Autodesk Inventor part; units mm, degrees
ref_plane "YZ Plane" through (0, 0, 0) normal (1, 0, 0) x (0, 1, 0)
ref_plane "XZ Plane" through (0, 0, 0) normal (0, 1, 0) x (-1, 0, 0)
ref_plane "XY Plane" through (0, 0, 0) normal (0, 0, 1) x (1, 0, 0)
sketch "Sketch1" plane through (0, 0, 0) normal (0, 1, 0) x (-1, 0, 0)
  line L0 (0, 0) -> (-21, 0)
  line L1 (-21, 0) -> (-21, -14)
  line L2 (-21, -14) -> (0, -14)
  line L3 (0, -14) -> (0, 0)
  dimension "d0" = 21
  dimension "d1" = 14
extrude "Extrusion1" add sketch "Sketch1" along normal blind 1.7
sketch "Sketch2" plane through (0, 0, 0) normal (0, -1, 0) x (1, 0, 0)
  line L0 (0, 0) -> (21, 0)
  line L1 (0, -14) -> (0, 0)
  line L2 (-4.6, 0) -> (27.6, 0)
  line L3 (0, -16.8) -> (0, 2.8)
  line L4 (0.52, -0.17) -> (6.02, -0.17)
  line L5 (6.02, -0.17) -> (6.02, -13.67)
  line L6 (6.02, -13.67) -> (0.52, -13.67)
  line L7 (0.52, -13.67) -> (0.52, -0.17)
  line L8 (2, -1.84) -> (2, -0.17)
  line L9 (2, -1.84) -> (0.52, -1.84)
  line L10 (4.54, -12) -> (4.54, -13.67)
  line L11 (4.54, -12) -> (6.02, -12)
  point P0 (4.54, -1.84)
  point P1 (2, -4.38)
  point P2 (4.54, -4.38)
  point P3 (2, -6.92)
  point P4 (4.54, -6.92)
  point P5 (2, -9.46)
  point P6 (4.54, -9.46)
  point P7 (2, -12)
  dimension "d12" = 2.54
  dimension "d15" = 2.54
  dimension "d18" = 5.5
  dimension "d19" = 13.5
  dimension "d20" = 4.38
  dimension "d21" = 4.54
extrude "Extrusion2" add sketch "Sketch2" along normal blind 9
sketch "Sketch3" plane through (0, 0, 0) normal (0, -1, 0) x (1, 0, 0)
  line L0 (0, -14) -> (0, 0)
  line L1 (13.1877, -8.8011) -> (20.6877, -8.8011)
  line L2 (20.6877, -8.8011) -> (20.6877, -0.3011)
  line L3 (20.6877, -0.3011) -> (13.1877, -0.3011)
  line L4 (13.1877, -0.3011) -> (13.1877, -8.8011)
  line L5 (19.1, -2.8011) -> (19.1, -0.3011)
  line L6 (19.1, -6.3011) -> (19.1, -8.8011)
  dimension "d25" = 19.1
  dimension "d26" = 3.5
  dimension "d27" = 7.5
  dimension "d28" = 8.5
extrude "Extrusion3" add sketch "Sketch3" along normal blind 13
properties part number "ccpad"
Design review of the part built by this model. Coordinates are the model's own, in mm. A direction names the side the tool comes from. Coordinates: 2 decimals unless noted, no trailing zeros. Write each loop counter-clockwise with the first axis right and the second up, starting at its lowest first coordinate (ties: lowest second). Pieces come first, ordered by that corner, then holes. Notation, with made-up numbers: M 41.25,46 L 99.25,46 A19 cw 99.25,57 Z; hole C 20,-6.5 d2. An arc over 180 degrees is marked long. Answer as a JSON object with one key per item and string values.
Item 1: Add section A-A, the plane y = -5.75. Give the boundary of the cut face in (x, z), and give its area (3 significant figures).
Outcome:
{"outline": "M 0.52,-13.67 L 6.02,-13.67 L 6.02,-0.17 L 0.52,-0.17 Z; M 13.19,-8.8 L 20.69,-8.8 L 20.69,-0.3 L 13.19,-0.3 Z", "area": "138 mm²"}
Item 2: Insertion check: pin 1 Ø2 at (y, z) = (-5, -5.5) entering from +X; pin 2 Ø1.5 at (x, z) = (3.5, -3.5) entering from -Y; pin 3 Ø2 at (x, y) = (15.5, -6) entering from -Z. Each pin has a flat end and moves straight along its axis. Give the tip position at first contact, or say it passes through.
Outcome:
{"pin 1": "x = 20.69", "pin 2": "y = -9", "pin 3": "z = -8.8"}
Item 3: Wall thickness on probe 1 along X at (y, z) = (-4.75, -6.5); probe 2 along Y at (x, z) = (3.75, -2); probe 3 along Z at (x, y) = (5.5, -3): over which ranges is each line inside the solid? List them lowest first.
Outcome:
{"probe 1": "0.52 to 6.02, 13.19 to 20.69", "probe 2": "-9 to 1.7", "probe 3": "-13.67 to -0.17"}
Item 4: Add section D-D, the plane z = -0.75. Give the boundary of the cut face in (x, y), and give its area (3 significant figures).
Outcome:
{"outline": "M 0,0 L 0.52,0 L 0.52,-9 L 6.02,-9 L 6.02,0 L 13.19,0 L 13.19,-13 L 20.69,-13 L 20.69,0 L 21,0 L 21,1.7 L 0,1.7 Z", "area": "183 mm²"}
Item 5: Machinability: for faces 5 (the flat face through (3, -4, -0.17)), 6 (the flat face through (13.188, -6, -4)), 7 (the flat face through (0.52, -4, -7)), 8 (the flat face through (17, -6, -8.801)), which of the approach directions +Z, -Z, +X, -X, +Y, -Y give a long, thin tool a straight path to every point of the face, cutting with its end or side? Answer none if there is none.
Outcome:
{"face 5": "+Z, +X, -X, -Y", "face 6": "+Z, -Z, -Y", "face 7": "+Z, -Z, -X, -Y", "face 8": "-Z, +X, -Y"}
Item 6: Draft analysis for pull direction X (two halves, no side actions). For faces 1 (the flat face through (6.02, -4, -7)), 2 (the flat face through (21, 1, -7)), 3 (the flat face through (0, 1, -7)), 4 (the flat face through (3, -4, -13.67)), state which applies: pulls with the +X half, pulls with the -X half, needs draft (parallel to the pull), parting line crosses it, or undercut.
Outcome:
{"face 1": "undercut", "face 2": "pulls with the +X half", "face 3": "pulls with the -X half", "face 4": "needs draft"}
Item 7: Add section C-C, the plane z = -10.25. Give the boundary of the cut face in (x, y).
Outcome:
{"outline": "M 0,0 L 0.52,0 L 0.52,-9 L 6.02,-9 L 6.02,0 L 21,0 L 21,1.7 L 0,1.7 Z"}
Item 8: Add section B-B, the plane x = 14.75. Give the boundary of the cut face in (y, z).
Outcome:
{"outline": "M -13,-8.8 L 0,-8.8 L 0,-14 L 1.7,-14 L 1.7,0 L 0,0 L 0,-0.3 L -13,-0.3 Z"}
